The model under review builds one solid part; all positions refer to its coordinate system, in mm. Round coordinates to 2 decimals unless told otherwise and drop trailing zeros. Order: outer loops, then holes, each group sorted by start corner. A loop starts at its lowest first (then second) coordinate and runs counter-clockwise, first axis right, second up. Notation, with made-up numbers: M 58,-0.75 L 70,-0.75 A20 ccw 70,33.25 Z; hole C 29.25,23.5 d1. An arc over 180 degrees is marked long. Use a Markdown table: item, result. Add a question column.
1. To check wall thickness, follow probe 1 along Y at (x, z) = (0, 0.9); probe 2 along X at (y, z) = (-59.18, 1.9) (3 decimals); probe 3 along X at (y, z) = (-9.5, 1.4). State the ranges of each line that lie inside material, in increasing order.
2. Insertion check: P1, Ø1.6, axis at y = -59.5, z = 1.5, coming from the -X side (3 decimals); P2, Ø1.5, axis at y = -0.5, z = 1.5, coming from the +X side; P3, Ø1.4, axis at x = 81, z = 2.5, coming from the +Y side. Each pin has a flat end and moves straight along its axis. Give the tip position at first contact, or say it passes through.
3. Consider section B-B on x = 55.5. State the section outline as (y, z) points.
4. Consider section A-A on z = 2. Count the separate pieces of the cut face and the enclosed holes in it, then the cut area to 3 significant figures.
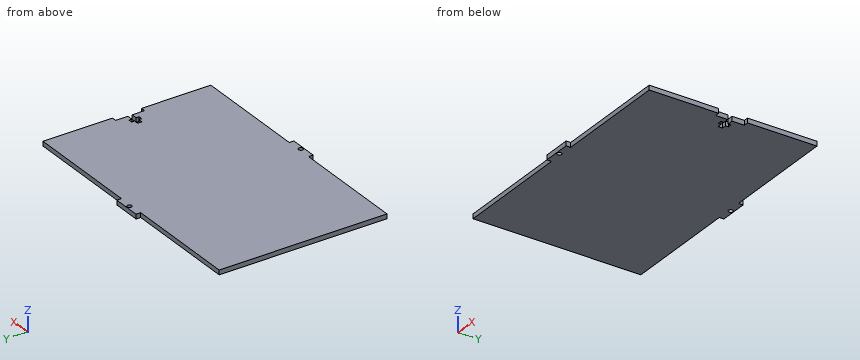
from build123d import *

# Parameters (mm, degrees)
SKETCH1_W               = 180
SKETCH1_H               = 122.36
BOSS_EXTRUDE1_DEPTH     = 3.18
CUT_EXTRUDE1_DEPTH      = 1
CUT_EXTRUDE1_DEPTH_BACK = 4.18
CUT_EXTRUDE2_START      = -4.18
SKETCH3_W               = 80.125
SKETCH3_H               = 3.18
CUT_EXTRUDE2_DEPTH      = 5.18
CUT_EXTRUDE3_START      = -4.18
SKETCH4_R               = 1.55
CUT_EXTRUDE3_DEPTH      = 5.18


with BuildPart() as part:
    # Sketch1 → Boss-Extrude1 (new body)
    with BuildSketch(Plane.XY):
        Rectangle(SKETCH1_W, SKETCH1_H)
    extrude(amount=BOSS_EXTRUDE1_DEPTH)

    # Sketch2 → Cut-Extrude1 (cut, two sides)
    with BuildSketch(Plane.XY.offset(3.18)) as cut_extrude1_sk:
        Polygon((80, 1.5), (77, 1.5), (77, -1.5), (80, -1.5), (80, -3.5), (82.82, -3.5), (82.82, -1.5), (86.82, -1.5), (86.82, -10), (90, -10), (90, 10), (86.82, 10), (86.82, 1.5), (82.82, 1.5), (82.82, 3.5), (80, 3.5), align=None)
    extrude(amount=CUT_EXTRUDE1_DEPTH, mode=Mode.SUBTRACT)
    extrude(cut_extrude1_sk.sketch, amount=-CUT_EXTRUDE1_DEPTH_BACK, mode=Mode.SUBTRACT)

    # Sketch3 → Cut-Extrude2 (cut)
    with BuildSketch(Plane.XY.offset(3.18).offset(CUT_EXTRUDE2_START)):
        with Locations((-49.9375, -59.59)):
            Rectangle(SKETCH3_W, SKETCH3_H)
        with Locations((49.9375, -59.59)):
            Rectangle(SKETCH3_W, SKETCH3_H)
    cut_extrude2 = extrude(amount=CUT_EXTRUDE2_DEPTH, mode=Mode.SUBTRACT)

    # Mirror1: Cut-Extrude2 across plane
    add(cut_extrude2.mirror(Plane.ZX), mode=Mode.SUBTRACT)

    # Sketch4 → Cut-Extrude3 (cut)
    with BuildSketch(Plane.XY.offset(3.18).offset(CUT_EXTRUDE3_START)):
        with Locations((0, -59.18)):
            Circle(SKETCH4_R)
    cut_extrude3 = extrude(amount=CUT_EXTRUDE3_DEPTH, mode=Mode.SUBTRACT)

    # Mirror2: Cut-Extrude3 across plane
    add(cut_extrude3.mirror(Plane.ZX), mode=Mode.SUBTRACT)


solid = part.part
Answer block:
| question | item | result |
|---|---|---|
| 1 | probe 1 | -61.18 to -60.73, -57.63 to 57.63, 60.73 to 61.18 |
| 1 | probe 2 | -9.875 to -1.55, 1.55 to 9.875 |
| 1 | probe 3 | -90 to 86.82 |
| 2 | P1 | x = -9.875 |
| 2 | P2 | x = 77 |
| 2 | P3 | y = 58 |
| 3 | outline | M -58,0 L 58,0 L 58,3.18 L -58,3.18 Z |
| 4 | separate pieces | 1 |
| 4 | enclosed holes | 2 |
| 4 | area | 20,900 mm^2 |
